Work out the finished part from the listing and answer in its coordinate system (mm). Round coordinates to 2 decimals unless told otherwise and drop trailing zeros. Write each loop counter-clockwise with the first axis right and the second up, starting at its lowest first coordinate (ties: lowest second). Pieces come first, ordered by that corner, then holes. Notation, with made-up numbers: (69, 32.25) -> (121, 32.25) arc R21 cw to (121, 59.25) -> close; hole circle Ø10 at (29, 38.25). An arc over 180 degrees is marked (long way). One line per question, with ' | ' between items. Start each with the question number.
```python
from build123d import *

# Parameters (mm, degrees)
BOSS_EXTRU_1_DEPTH           = 3.5
ESQUISSE2_R                  = 2
ENL_V_MAT_EXTRU_1_DEPTH      = 395.382111663
ESQUISSE3_R                  = 2
ENL_V_MAT_EXTRU_2_DEPTH      = 395.382111663
ENL_V_MAT_EXTRU_3_DEPTH      = 395.382111663
ENL_V_MAT_EXTRU_4_DEPTH      = 395.382111663
ENL_V_MAT_EXTRU_4_DEPTH_BACK = 395.382111663
ESQUISSE6_R                  = 1.5
ENL_V_MAT_EXTRU_5_DEPTH      = 309.078317965
CONG_1_R                     = 5
ESQUISSE7_R                  = 37.5
ENL_V_MAT_EXTRU_6_DEPTH      = 309.078317965


with BuildPart() as part:
    # Esquisse1 → Boss.-Extru.1 (new body)
    with BuildSketch(Plane.XY):
        with BuildLine():
            Line((5, 0), (245, 0))
            ThreePointArc((245, 0), (248.535533906, 1.464466094), (250, 5))
            Line((250, 5), (250, 305))
            Line((250, 305), (0, 305))
            Line((0, 305), (0, 5))
            ThreePointArc((0, 5), (1.464466094, 1.464466094), (5, 0))
        make_face()
    extrude(amount=BOSS_EXTRU_1_DEPTH)

    # Esquisse2 → Enlèv. mat.-Extru.1 (cut, through all)
    with BuildSketch(Plane.XY.offset(3.5)):
        with Locations((5, 5)):
            Circle(ESQUISSE2_R)
        with Locations((245, 5)):
            Circle(ESQUISSE2_R)
        with Locations((5, 58.8)):
            Circle(ESQUISSE2_R)
        with Locations((245, 58.8)):
            Circle(ESQUISSE2_R)
    extrude(amount=-ENL_V_MAT_EXTRU_1_DEPTH, mode=Mode.SUBTRACT)

    # Esquisse3 → Enlèv. mat.-Extru.2 (cut, through all)
    with BuildSketch(Plane.XY.offset(3.5)):
        with Locations((57, 5)):
            Circle(ESQUISSE3_R)
        with Locations((193, 5)):
            Circle(ESQUISSE3_R)
    extrude(amount=-ENL_V_MAT_EXTRU_2_DEPTH, mode=Mode.SUBTRACT)

    # Esquisse4 → Enlèv. mat.-Extru.3 (cut, through all)
    with BuildSketch(Plane(origin=(0, 0, 0), x_dir=(-1, 0, 0), z_dir=(0, 0, -1))):
        with BuildLine():
            Line((-70, 15), (-70, 50))
            ThreePointArc((-70, 50), (-68.535533906, 53.535533906), (-65, 55))
            Line((-65, 55), (-15, 55))
            ThreePointArc((-15, 55), (-11.464466094, 53.535533906), (-10, 50))
            Line((-10, 50), (-10, 15))
            ThreePointArc((-10, 15), (-11.464466094, 11.464466094), (-15, 10))
            Line((-15, 10), (-65, 10))
            ThreePointArc((-65, 10), (-68.535533906, 11.464466094), (-70, 15))
        make_face()
        with BuildLine():
            Line((-185, 10), (-235, 10))
            ThreePointArc((-235, 10), (-238.535533906, 11.464466094), (-240, 15))
            Line((-240, 15), (-240, 50))
            ThreePointArc((-240, 50), (-238.535533906, 53.535533906), (-235, 55))
            Line((-235, 55), (-185, 55))
            ThreePointArc((-185, 55), (-181.464466094, 53.535533906), (-180, 50))
            Line((-180, 50), (-180, 15))
            ThreePointArc((-180, 15), (-181.464466094, 11.464466094), (-185, 10))
        make_face()
    extrude(amount=-ENL_V_MAT_EXTRU_3_DEPTH, mode=Mode.SUBTRACT)

    # Esquisse5 → Enlèv. mat.-Extru.4 (cut, two sides: drawn at the far end of the back side and taken through both)
    with BuildSketch(Plane.XY.offset(3.5).offset(-ENL_V_MAT_EXTRU_4_DEPTH_BACK)):
        Polygon((-374.383398967, -414.136758554), (0, 110), (50, 180), (200, 180), (250, 110), (624.383398967, -414.136758554), (624.383398967, 874.090350445), (-374.383398967, 874.090350445), align=None)
    extrude(amount=ENL_V_MAT_EXTRU_4_DEPTH + ENL_V_MAT_EXTRU_4_DEPTH_BACK, mode=Mode.SUBTRACT)

    # Esquisse6 → Enlèv. mat.-Extru.5 (cut, through all)
    with BuildSketch(Plane.XY.offset(3.5)):
        with Locations((125, 166)):
            Circle(ESQUISSE6_R)
    extrude(amount=-ENL_V_MAT_EXTRU_5_DEPTH, mode=Mode.SUBTRACT)

    # Congé1
    cong_1_edges = [part.edges().sort_by_distance(p)[0] for p in [
        (50, 180, 1.75),
        (200, 180, 1.75),
        (250, 110, 1.75),
        (0, 110, 1.75),
    ]]
    fillet(cong_1_edges, radius=CONG_1_R)

    # Esquisse7 → Enlèv. mat.-Extru.6 (cut, through all)
    with BuildSketch(Plane.XY.offset(3.5)):
        with Locations((59.6, 104.646798594)):
            Circle(ESQUISSE7_R)
    extrude(amount=-ENL_V_MAT_EXTRU_6_DEPTH, mode=Mode.SUBTRACT)


solid = part.part
```
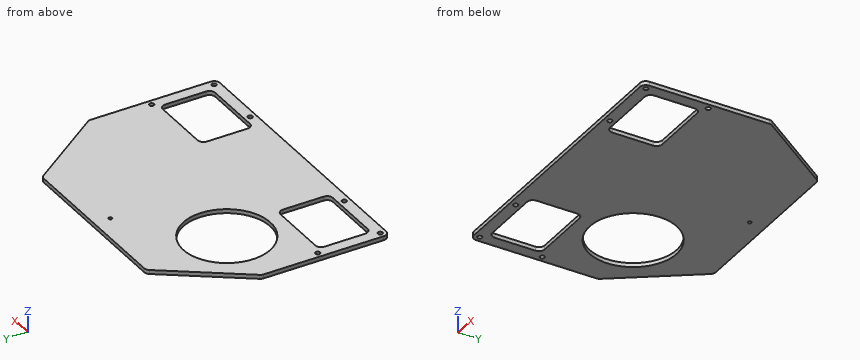
(1) Given pin 1 Ø3 at (x, y) = (57, 5) entering from -Z; pin 2 Ø1 at (x, z) = (42.5, 1.5) entering from +Y; pin 3 Ø1.8 at (x, z) = (200, 2) entering from +Y, each flat-ended and moving along its own axis, determine where each tip first touches the part or whether it passes through.
(2) Consider L1, parallel to X at y = 48.5, z = 3.05; L2, parallel to X at y = 58.5, z = 2.9; L3, parallel to Y at x = 125, z = 2. Determine where each line is inside the solid, lowest interval first.
(3) A cutting plane is placed at C-C, the plane z = 1.4. Count the separate pieces of the cut face and the enclosed holes in it, then the cut area to 3 significant figures.
(4) A cutting plane is placed at B-B, the plane x = 88.5. Determine the outline of the cut face in (y, z).
(5) A cutting plane is placed at A-A, the plane x = 19. Determine the outline of the cut face in (y, z).
Returned:
1) pin 1: through | pin 2: y = 170.2 | pin 3: y = 179.71
2) L1: 0 to 10, 70 to 180, 240 to 250 | L2: 0 to 3.02, 6.98 to 243.02, 246.98 to 250 | L3: 0 to 164.5, 167.5 to 180
3) separate pieces: 1 | enclosed holes: 10 | area: 31,600 mm2
4) outline: (0, 0) -> (80.75, 0) -> (80.75, 3.5) -> (0, 3.5) -> close; (128.54, 0) -> (180, 0) -> (180, 3.5) -> (128.54, 3.5) -> close
5) outline: (0, 0) -> (10, 0) -> (10, 3.5) -> (0, 3.5) -> close; (55, 0) -> (136.6, 0) -> (136.6, 3.5) -> (55, 3.5) -> close
